Autodesk Inventor part; units mm, degrees
ref_plane "YZ Plane" through (0, 0, 0) normal (1, 0, 0) x (0, 1, 0)
ref_plane "XZ Plane" through (0, 0, 0) normal (0, 1, 0) x (-1, 0, 0)
ref_plane "XY Plane" through (0, 0, 0) normal (0, 0, 1) x (1, 0, 0)
sketch "Sketch1" plane through (0, 0, 0) normal (0, 0, 1) x (1, 0, 0)
  circle A0 centre (15.9889, 3.0332) radius 69.85 construction
  line L0 (85.8389, 3.0332) -> (50.9139, -57.4587) construction
  line L1 (50.9139, -57.4587) -> (-18.9361, -57.4587) construction
  line L2 (-18.9361, -57.4587) -> (-53.8611, 3.0332) construction
  line L3 (-53.8611, 3.0332) -> (-18.9361, 63.5251) construction
  line L4 (-18.9361, 63.5251) -> (50.9139, 63.5251) construction
  line L5 (50.9139, 63.5251) -> (85.8389, 3.0332) construction
  line L6 (85.8389, 3.0332) -> (85.8389, 780.9082) construction
  line L7 (85.8389, 3.0332) -> (85.8389, 3.0332) construction
  line L8 (-53.8611, 3.0332) -> (85.8389, 3.0332) construction
  arc A1 (85.8389, 780.9082) -> (-303.0986, 676.6927) centre (85.8389, 3.0332) ccw
  arc A2 (-303.0986, 676.6927) -> (-657.1111, 63.5251) centre (50.9139, 63.5251) ccw
  arc A3 (-657.1111, 63.5251) -> (-338.0236, -489.1507) centre (-18.9361, 63.5251) ccw
  arc A4 (-338.0236, -489.1507) -> (230.3014, -489.1507) centre (-53.8611, 3.0332) ccw
  arc A5 (230.3014, -489.1507) -> (479.5389, -57.4587) centre (-18.9361, -57.4587) ccw
  line L9 (85.8389, 780.9082) -> (587.4889, 780.9082)
  circle A6 centre (435.5017, 175.6262) radius 21.082 construction
  line L10 (50.9139, -57.4587) -> (435.5017, 175.6262) construction
  line L11 (85.8389, 784.0832) -> (587.4889, 784.0832)
  arc A7 (85.8389, 784.0832) -> (-304.6861, 679.4423) centre (85.8389, 3.0332) ccw
  arc A8 (-304.6861, 679.4423) -> (-660.2861, 63.5251) centre (50.9139, 63.5251) ccw
  arc A9 (-660.2861, 63.5251) -> (-339.6111, -491.9003) centre (-18.9361, 63.5251) ccw
  arc A10 (-339.6111, -491.9003) -> (231.8889, -491.9003) centre (-53.8611, 3.0332) ccw
  arc A11 (231.8889, -491.9003) -> (482.7139, -57.4587) centre (-18.9361, -57.4587) ccw
  line L12 (587.4889, 784.0832) -> (587.4889, 780.9082)
  line L13 (15.9889, 72.8832) -> (15.9889, -66.8168) construction
  line L14 (425.7203, 156.9507) -> (423.0042, 155.3045)
  arc A12 (482.7139, -57.4587) -> (425.7203, 156.9507) centre (50.9139, -57.4587) ccw
  arc A13 (479.5389, -57.4587) -> (423.0042, 155.3045) centre (50.9139, -57.4587) ccw
  arc A14 (423.0042, 155.3045) -> (417.4725, 164.6993) centre (50.9139, -57.4587) ccw construction
  dimension "d2" = 42.164
  dimension "d1" = 777.875
  dimension "d3" = 172.593
  dimension "d5" = 449.707
  dimension "d6" = 3.175
  dimension "d8" = 571.5
  dimension "d9" = 428.625
extrude "Extrusion1" add sketch "Sketch1" along normal blind 447.675
ref_plane "Work Plane1" through (587.4889, 784.0832, 223.8375) normal (0, 0, 1) x (1, 0, 0)
equation "\"d5\" = d4 + 0.5 * d2"
equation "\"BendRadius\" = Thickness"
equation "\"BendReliefWidth\" = Thickness"
equation "\"BendReliefDepth\" = 0.5 * Thickness"
equation "\"CornerReliefSize\" = 4 * Thickness"
equation "\"MinimumRemnant\" = 2 * Thickness"
equation "\"TransitionRadius\" = BendRadius"
equation "\"JacobiRadiusSize\" = Thickness"
equation "\"GapSize\" = Thickness"
properties part number "band" material "Steel, Mild"
The model under review builds one solid part; all positions refer to its coordinate system, in mm. A direction names the side the tool comes from. Coordinates: 2 decimals unless noted, no trailing zeros. Loops run counter-clockwise (first coordinate to the right, second up) from the corner with the lowest first, then second, coordinate; pieces in that order, holes last. Notation, with made-up numbers: (55, 35.25) -> (96, 35.25) arc R15 cw to (96, 63.25) -> close; hole circle Ø2 at (15.25, -33). An arc over 180 degrees is marked (long way). Answer as CSV lines item,"result".
Item 1: Insertion check: pin 1 (3 mm diameter, centred on x = -332, z = 93, fed in from +Y); pin 2 (2 mm diameter, centred on x = 376, z = 370, fed in from -Y); pin 3 (1 mm diameter, centred on y = -130.5, z = 370.5, fed in from +X). Each pin has a flat end and moves straight along its axis. Give the tip position at first contact, or say it passes through.
Results below:
pin 1,"stops at y = 663.8"
pin 2,"stops at y = -368.05"
pin 3,"stops at x = 477.44"
Item 2: For L1, parallel to Y at x = -431.5, z = 25; L2, parallel to Y at x = -217.5, z = 168; L3, parallel to X at y = -388.5, z = 33, list the stretches that pass through material, from the lowest coordinate up.
Results below:
L1,"y = -427.52 to -423.36, 581.77 to 586.1"
L2,"y = -544.54 to -541.22, 719.33 to 722.77"
L3,"x = -473.91 to -469.43, 353.74 to 357.98"
Item 3: Take a section at A-A, the plane x = -530.5. State the section outline as (y, z) points (3 decimals), and give its area (3 significant figures).
Results below:
outline,"(-323.298, 0) -> (-318.011, 0) -> (-318.011, 447.675) -> (-323.298, 447.675) -> close; (467.576, 0) -> (473.114, 0) -> (473.114, 447.675) -> (467.576, 447.675) -> close"
area,"4,850 mm2"
Item 4: Draft analysis for pull direction X (two halves, no side actions). For faces 4 (the cylindrical face through (464.76, 54.12, 220.7)), 5 (the cylindrical face through (467.816, 54.986, 220.704)), 6 (the cylindrical face through (-49.695, -565.277, 220.704)), 7 (the cylindrical face through (-119.076, 756.724, 220.704)), state which applies: +X half, -X half, draft (parallel to the pull), parting line (faces both ways), or undercut.
Results below:
face 4,"undercut"
face 5,"+X half"
face 6,"undercut"
face 7,"-X half"
Item 5: Take a section at C-C, the plane z = 50. State the section outline as (x, y) points, and give its area (3 significant figures).
Results below:
outline,"(-660.29, 63.53) arc R641.35 ccw to (-339.61, -491.9) arc R571.5 ccw to (231.89, -491.9) arc R501.65 ccw to (482.71, -57.46) arc R431.8 ccw to (425.72, 156.95) -> (423, 155.3) arc R428.62 cw to (479.54, -57.46) arc R498.48 cw to (230.3, -489.15) arc R568.33 cw to (-338.02, -489.15) arc R638.18 cw to (-657.11, 63.53) arc R708.03 cw to (-303.1, 676.69) arc R777.87 cw to (85.84, 780.91) -> (587.49, 780.91) -> (587.49, 784.08) -> (85.84, 784.08) arc R781.05 ccw to (-304.69, 679.44) arc R711.2 ccw to start"
area,"11,600 mm2"
Item 6: Machinability: for faces 1 (the cylindrical face through (-569.258, -259.605, 220.704)), 2 (the flat face through (333, 784.083, 221)), 3 (the cylindrical face through (-118.24, 753.66, 220.7)), which of the approach directions +Z, -Z, +X, -X, +Y, -Y give a long, thin tool a straight path to every point of the face, cutting with its end or side? Answer none if there is none.
Results below:
face 1,"+Z, -Z"
face 2,"+Z, -Z, +X, -X, +Y"
face 3,"+Z, -Z, +X"
